Here's the drawing with two shaded views (mm, measured from the low corner). I have some questions. Give positions to 0.01 mm unless a question says otherwise; leave off trailing zeros. Order: outer loops, then holes, each group sorted by start corner. A loop starts at its lowest first (then second) coordinate and runs counter-clockwise, first axis right, second up. Notation, with made-up numbers: (11.25, 19.5) - (49.25, 19.5) arc R27 ccw to (49.25, 35.5) - close; hole circle Ø11 at (-24, -12.5). An arc over 180 degrees is marked (long way). Use one line per item in the form item = value. Start each with the question number.
1) Suppose I cut it at C-C, the plane x = 42.5. Write out the boundary of the cut face in (y, z), and give its area (3 significant figures).
2) Suppose I cut it at A-A, the plane y = 12.5. Write out the boundary of the cut face in (x, z).
3) Suppose I cut it at B-B, the plane z = 15.5. Write out the boundary of the cut face in (x, y).
4) We'd pull the mould along X, two halves only. Please class the marked faces 1, 2 and 3: released by +X, released by -X, zero draft, split by the parting line, or undercut.
5) Please list where these lines run through material, in increasing order: probe 1 along X at (y, z) = (12.75, 69); probe 2 along Y at (x, z) = (6.5, 70).
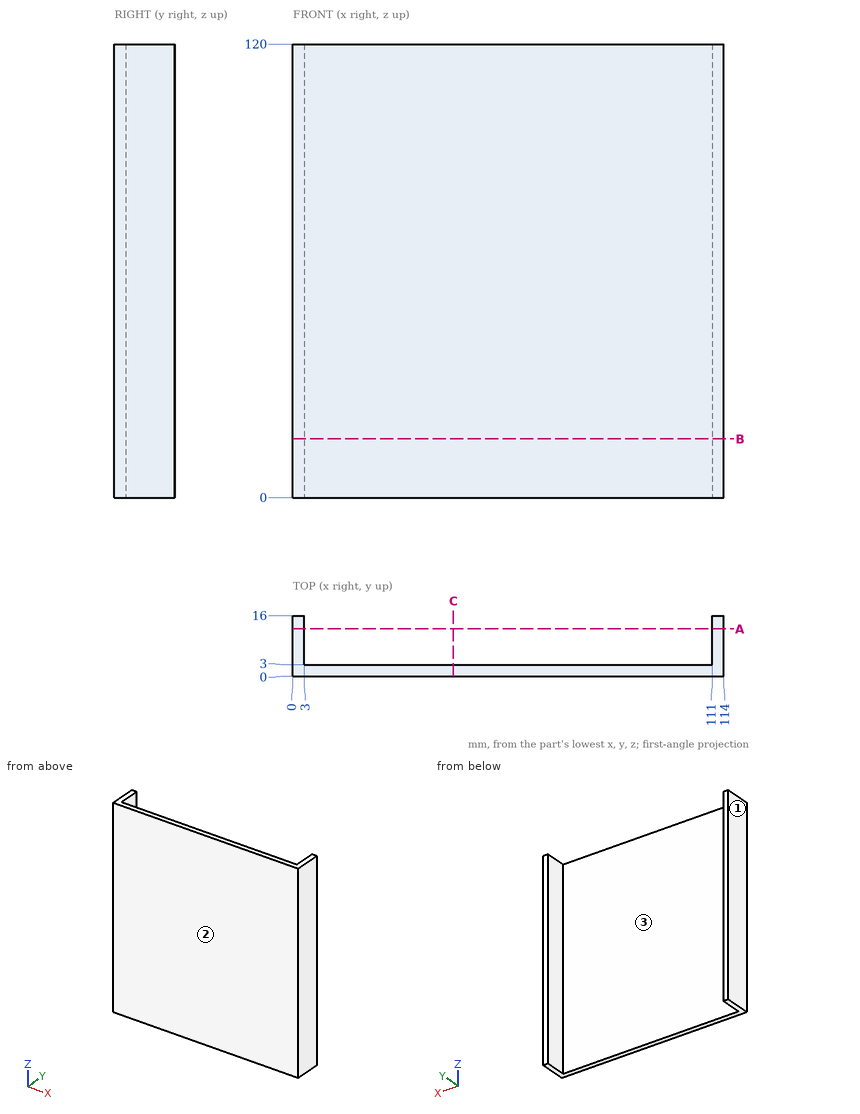
Result sheet:
q1.outline = (0, 0) - (3, 0) - (3, 120) - (0, 120) - close
q1.area = 360 mm²
q2.outline = (0, 0) - (3, 0) - (3, 120) - (0, 120) - close; (111, 0) - (114, 0) - (114, 120) - (111, 120) - close
q3.outline = (0, 0) - (114, 0) - (114, 16) - (111, 16) - (111, 3) - (3, 3) - (3, 16) - (0, 16) - close
q4.face_1 = released by -X
q4.face_2 = zero draft
q4.face_3 = undercut
q5.probe_1 = 0 to 3, 111 to 114
q5.probe_2 = 0 to 3
